Job drawing, mm, ordinate dimensions from the low corner. One solid piece. Round coordinates to 2 decimals unless told otherwise and drop trailing zeros. Loops run counter-clockwise (first coordinate to the right, second up) from the corner with the lowest first, then second, coordinate; pieces in that order, holes last.
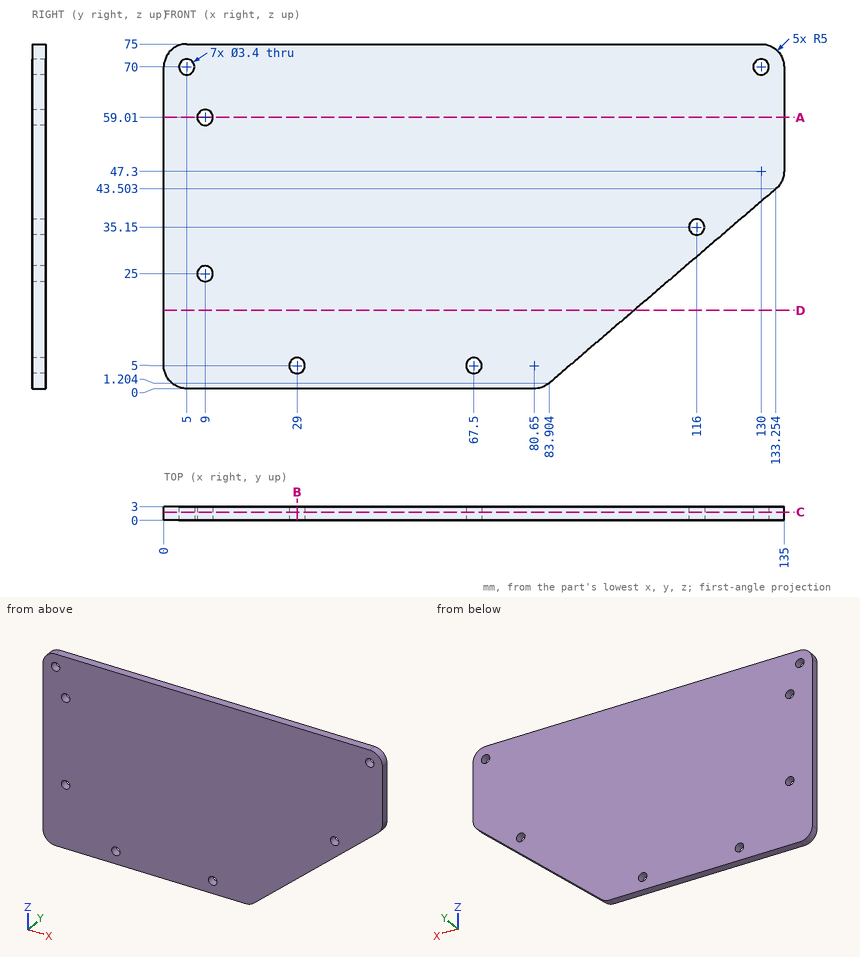
1) Slice it at C-C, the plane y = 1.8. Give the number of separate pieces and of enclosed holes in the cut face, then the cut area to 3 significant figures.
Values:
separate pieces: 1
enclosed holes: 7
area: 8,860 mm2
2) Slice it at B-B, the plane x = 29. Give the cut face in (y, z).
Values:
outline: (0, 0) - (3, 0) - (3, 3.3) - (0, 3.3) - close; (0, 6.7) - (3, 6.7) - (3, 75) - (0, 75) - close
3) Slice it at A-A, the plane z = 59.01. Give the cut face in (x, y).
Values:
outline: (0, 0) - (7.3, 0) - (7.3, 3) - (0, 3) - close; (10.7, 0) - (135, 0) - (135, 3) - (10.7, 3) - close
4) Slice it at D-D, the plane z = 17. Give the cut face in (x, y).
Values:
outline: (0, 0) - (102.33, 0) - (102.33, 3) - (0, 3) - close
5) Wall check: line 1 along Z through (x, y) = (9, 1.8); line 2 along Z through (x, y) = (10, 2.25) (1 decimal); line 3 along Z through (x, y) = (29, 1.45). Give the ranges that are in metal, low to high.
Values:
line 1: z = 0 to 23.3, 26.7 to 57.31, 60.71 to 75
line 2: z = 0 to 23.6, 26.4 to 57.6, 60.4 to 75
line 3: z = 0 to 3.3, 6.7 to 75
6) Drop a flat-ended pin along its axis: pin 1 Ø1 at (y, z) = (1.5, 22.5) entering from +X (1 decimal). Give the stop position or say it passes through.
Values:
pin 1: stops at x = 109.3
